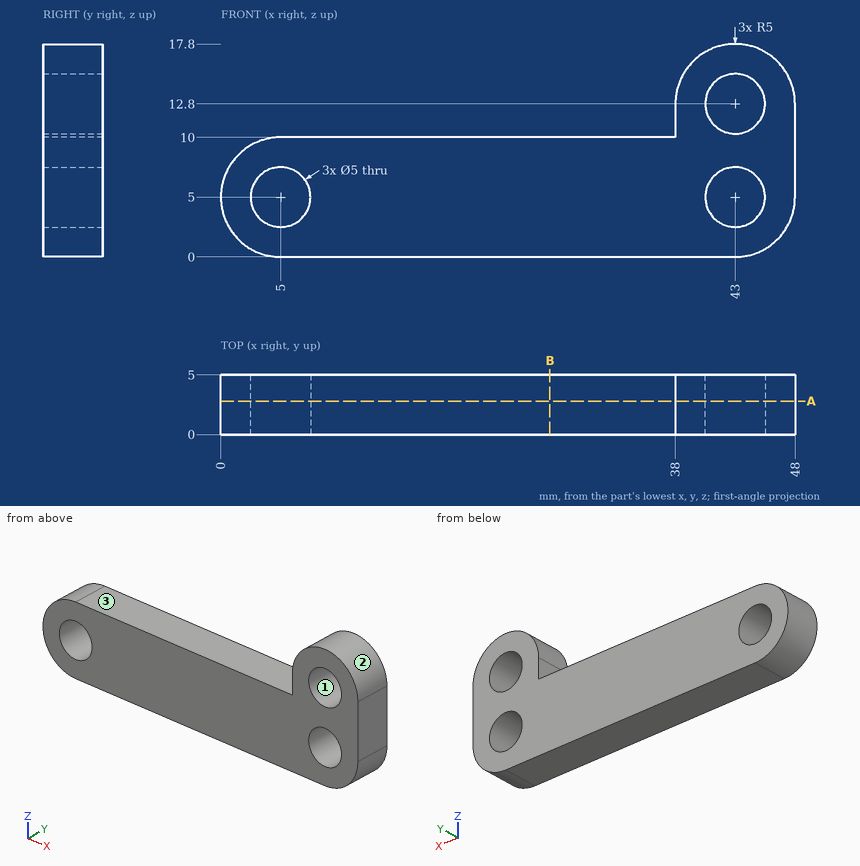
Job drawing, mm, ordinate dimensions from the low corner. One solid piece. Coordinates: 2 decimals unless noted, no trailing zeros. Loops run counter-clockwise (first coordinate to the right, second up) from the corner with the lowest first, then second, coordinate; pieces in that order, holes last. Notation, with made-up numbers: (-16, -29) - (1, -29) arc R31 cw to (1, 2) - close; hole circle Ø11 at (1, -35.5). An arc over 180 degrees is marked (long way). Write item = value, one per line. Start each with the question number.
Q1. Flat gauge pins, fed straight in: pin 1 Ø1.5 at (x, y) = (16, 3) entering from +Z; pin 2 Ø4 at (x, z) = (43, 5) entering from -Y; pin 3 Ø3 at (y, z) = (2.5, 12) entering from -X; pin 4 Ø3 at (x, y) = (39.5, 1.5) entering from +Z. Where does each tip first touch, or does it go through?
Q2. Drill centre lines: L1, parallel to Z at x = 43, y = 2.7; L2, parallel to X at y = 2.25, z = 4.25; L3, parallel to Z at x = 5, y = 2.2. Where is each one in solid material? Low to high.
Q3. Pull direction X, two halves, no side cores. Call the marked faces 1, 2 and 3: pulls with the +X half, pulls with the -X half, needs draft (parallel to the pull), parting line crosses it, or undercut.
Q4. Cut at A-A, the plane y = 2.8. List the corners of the cut face in (x, z).
Q5. Cut at B-B, the plane x = 27.5. List the corners of the cut face in (y, z).
Computed:
q1.pin_1 = 10
q1.pin_2 = through
q1.pin_3 = 38
q1.pin_4 = 17.38
q2.L1 = 0 to 2.5, 7.5 to 10.3, 15.3 to 17.8
q2.L2 = 0.06 to 2.62, 7.38 to 40.62, 45.38 to 47.94
q2.L3 = 0 to 2.5, 7.5 to 10
q3.face_1 = undercut
q3.face_2 = parting line crosses it
q3.face_3 = needs draft
q4.outline = (5, 0) - (43, 0) arc R5 ccw to (48, 5) - (48, 12.8) arc R5 ccw to (38, 12.8) - (38, 10) - (5, 10) arc R5 ccw to start; hole circle Ø5 at (5, 5); hole circle Ø5 at (43, 5); hole circle Ø5 at (43, 12.8)
q5.outline = (0, 0) - (5, 0) - (5, 10) - (0, 10) - close
